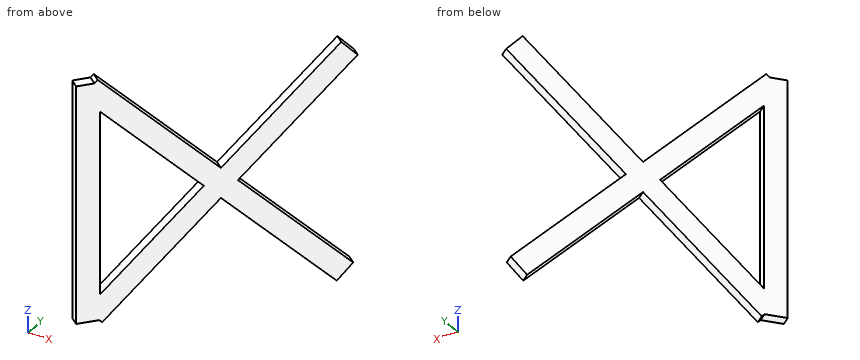
from build123d import *

# Parameters (mm, degrees)
BOX238_W                  = 0.5
BOX238_H                  = 1
BOX238_DEPTH              = 15
BOX238_ROLL_ANGLE         = 46
BOX239_W                  = 0.5
BOX239_H                  = 1
BOX239_DEPTH              = 15
BOX239_ROLL_ANGLE         = -46
BOX237_W                  = 0.5
BOX237_H                  = 1
BOX237_DEPTH              = 11
FUSION022_PLACEMENT_ANGLE = -39.8


with BuildPart() as cubo238:
    # Box238 → Box238 (new body)
    with BuildSketch(Plane.XY):
        with Locations((0.25, 0.5)):
            Rectangle(BOX238_W, BOX238_H)
    extrude(amount=BOX238_DEPTH)


with BuildPart() as cubo238_1:
    # Box238 roll: moved
    add(cubo238.part.rotate(Axis((0, 0, 0), (1, 0, 0)), BOX238_ROLL_ANGLE))


with BuildPart() as cubo238_2:
    # Box238 placement: moved
    add(cubo238_1.part.moved(Location((0, 11, 0.5))))


with BuildPart() as cubo239:
    # Box239 → Box239 (new body)
    with BuildSketch(Plane.XY):
        with Locations((0.25, 0.5)):
            Rectangle(BOX239_W, BOX239_H)
    extrude(amount=BOX239_DEPTH)


with BuildPart() as cubo239_1:
    # Box239 roll: moved
    add(cubo239.part.rotate(Axis((0, 0, 0), (1, 0, 0)), BOX239_ROLL_ANGLE))


with BuildPart() as cubo239_2:
    # Box239 placement: moved
    add(cubo239_1.part.moved(Location((0, 0.4, 1.1))))


with BuildPart() as fusion022:
    # Box237 → Box237 (new body)
    with BuildSketch(Plane.XY.offset(0.5)):
        with Locations((0.25, 0.5)):
            Rectangle(BOX237_W, BOX237_H)
    extrude(amount=BOX237_DEPTH)

    # Fusion022: union Cubo238, Cubo239
    add(cubo238_2.part)
    add(cubo239_2.part)


with BuildPart() as fusion022_1:
    # Fusion022 placement: moved
    add(fusion022.part.moved(Location((-178.9, 150.89, 0))).rotate(Axis((-178.9, 150.89, 0), (0, 0, 1)), FUSION022_PLACEMENT_ANGLE))


solid = fusion022_1.part
Design review of the part built by this model. Coordinates are the model's own, in mm. Round coordinates to 2 decimals unless told otherwise and drop trailing zeros. Write each loop counter-clockwise with the first axis right and the second up, starting at its lowest first coordinate (ties: lowest second). Pieces come first, ordered by that corner, then holes. Notation, with made-up numbers: M 21,58 L 65,58 A36 cw 65,97 Z; hole C 53,8 d4. An arc over 180 degrees is marked long. One line per item, written item: value. Start each with the question number.
1. Clearance check with flat-ended pins moving along their axes: P1, Ø1.5, axis at y = 153.5, z = 6.5, coming from the +X side; P2, Ø1.1, axis at x = -178.5, y = 151, coming from the -Z side; P3, Ø1.5, axis at x = -175.5, z = 7.5, coming from the +Y side. State where each tip first meets the part, or that it passes through.
2. Take a section at C-C on z = 9.5. State the section outline as (x, y) points.
3. Take a section at D-D on x = -174.75. State the section outline as (y, z) points, then the cut area to 3 significant figures.
4. Take a section at A-A on z = 1. State the section outline as (x, y) points.
5. To check wall thickness, follow probe 1 along X at (y, z) = (157, 3.5); probe 2 along X at (y, z) = (158.75, 9.75); probe 3 along Y at (x, z) = (-177, 10). State the ranges of each line that lie inside material, in increasing order. Write a range as from..to.
6. Take a section at B-B on y = 152.25. State the section outline as (x, z) points.
Computed:
1. P1: stops at x = -175.45
1. P2: stops at z = 0.5
1. P3: stops at y = 155.4
2. outline: M -178.9,150.89 L -178.52,150.57 L -177.88,151.34 L -178.26,151.66 Z; M -177.82,152.18 L -177.44,151.86 L -176.52,152.97 L -176.9,153.29 Z; M -173.08,157.88 L -172.69,157.56 L -171.77,158.67 L -172.15,158.99 Z
3. outline: M 155.09,5 L 155.38,5.22 L 155.87,4.86 L 155.87,6.97 L 155.38,6.61 L 155.09,6.83 Z
3. area: 1.33 mm²
4. outline: M -178.9,150.89 L -178.52,150.57 L -177.4,151.9 L -177.79,152.22 Z; M -172.19,158.94 L -171.81,158.62 L -171.17,159.39 L -171.55,159.71 Z
5. probe 1: x = -173.81..-173.16
5. probe 2: x = -172.35..-171.7
5. probe 3: y = 152.39..152.69
6. outline: M -177.77,1.03 L -177.12,1.44 L -177.12,2.83 L -177.77,2.42 Z; M -177.77,9.41 L -177.12,9.01 L -177.12,10.4 L -177.77,10.8 Z
